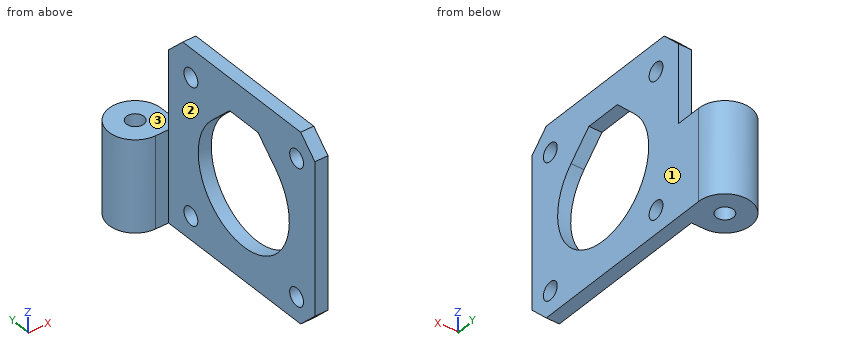
```python
from build123d import *

# Parameters (mm, degrees)
BOX_W        = 2.5
BOX_H        = 36
BOX_DEPTH    = 36
SKETCH_R     = 1.65
PAD_DEPTH    = 17.5
SKETCH001_R  = 1.7
POCKET_DEPTH = 5
CHAMFER_SIZE = 3.5


with BuildPart() as cubo:
    # Box → Box (new body)
    with BuildSketch(Plane.XY):
        with Locations((1.25, 18)):
            Rectangle(BOX_W, BOX_H)
    extrude(amount=BOX_DEPTH)


with BuildPart() as chamfer_body:
    # Sketch → Pad (new body)
    with BuildSketch(Plane.XY):
        with BuildLine():
            Line((0, 0), (2.5, 0))
            Line((2.5, 0), (2.5, 36))
            Line((2.5, 36), (5.000024, 36))
            ThreePointArc((5.000024, 36), (8.535534, 44.535534), (0, 41.000023))
            Line((0, 41.000023), (0, 0))
        make_face()
        with Locations((5, 41)):
            Circle(SKETCH_R, mode=Mode.SUBTRACT)
    extrude(amount=PAD_DEPTH)

    # Fusion: union Cubo
    add(cubo.part)

    # Sketch001 → Pocket (cut)
    with BuildSketch(Plane.YZ.offset(2.5)):
        with Locations((4.5, 30.5)):
            Circle(SKETCH001_R)
        with Locations((30.5, 30.5)):
            Circle(SKETCH001_R)
        with Locations((30.5, 4.5)):
            Circle(SKETCH001_R)
        with Locations((4.5, 4.5)):
            Circle(SKETCH001_R)
        with BuildLine():
            Line((9.580377, 25.419569), (14, 29.839192))
            Line((14, 29.839192), (21, 29.839192))
            Line((21, 29.839192), (25.419623, 25.419569))
            ThreePointArc((9.580377, 25.419569), (17.5, 6.3), (25.419623, 25.419569))
        make_face()
    extrude(amount=-POCKET_DEPTH, mode=Mode.SUBTRACT)

    # Chamfer
    chamfer_edges = [chamfer_body.edges().sort_by_distance(p)[0] for p in [
        (1.25, 36, 36),
        (1.25, 0, 36),
        (1.25, 0, 0),
    ]]
    chamfer(chamfer_edges, length=CHAMFER_SIZE)


with BuildPart() as part_mirroring:
    # Part__Mirroring: instance of Chamfer body
    add(chamfer_body.part.mirror(Plane(origin=(0, 0, 0), x_dir=(0, -1, 0), z_dir=(1, 0, 0))))


solid = part_mirroring.part
```
The listing builds one solid part. Answer for the finished solid, in the listing's coordinates (mm). Face numbers are marked on the shaded views. A direction names the side the tool comes from. Coordinates: 2 decimals unless noted, no trailing zeros. Write each loop counter-clockwise with the first axis right and the second up, starting at its lowest first coordinate (ties: lowest second). Pieces come first, ordered by that corner, then holes. Notation, with made-up numbers: (45, 67.25) -> (99, 67.25) arc R16 ccw to (99, 84.25) -> close; hole circle Ø6 at (87.5, 50.25). An arc over 180 degrees is marked (long way). Write each question's results on one line, items separated by ' | '. Start each with the question number.
1) Straight lines are drawn through the part: probe 1 along Z at (x, y) = (-1.55, 4.5); probe 2 along Z at (x, y) = (-1.95, 17.5); probe 3 along Y at (x, z) = (-1.5, 3.5). For each, find the intervals that lie inside material, in ascending order.
2) A cutting plane is placed at A-A (z = 4.5). Determine the outline of the cut face in (x, y), then the cut area to 3 significant figures.
3) Flat-ended cylindrical pins translate along their axes: pin 1 Ø3 at (x, y) = (-6.5, 40) entering from +Z; pin 2 Ø20 at (y, z) = (17.5, 17.5) entering from +X; pin 3 Ø4.5 at (y, z) = (4.5, 30.5) entering from -X; pin 4 Ø3 at (x, z) = (-0.5, 26) entering from +Y. Find the tip coordinate at first contact, or state that the pin passes through.
4) A cutting plane is placed at C-C (y = 30.5). Determine the outline of the cut face in (x, z), then the cut area to 3 significant figures.
5) A cutting plane is placed at D-D (x = -2). Determine the outline of the cut face in (y, z).
6) A tool of negligible diameter and unlimited length cuts with its end or side. For the marked faces 1, 2 and 3, from which of +Z, -Z, +X, -X, +Y, -Y can it reach the whole face along a straight path? Write none if from no direction.
7) A cutting plane is placed at B-B (z = 14). Determine the outline of the cut face in (x, y).
Values follow:
1) probe 1: 0 to 2.8, 6.2 to 28.8, 32.2 to 36 | probe 2: 0 to 6.3, 29.84 to 36 | probe 3: 0 to 3.13, 5.87 to 29.13, 31.87 to 44.57
2) outline: (-5, 36) -> (-2.5, 36) -> (-2.5, 32.2) -> (0, 32.2) -> (0, 41) arc R5 ccw (long way) to start; (-2.5, 0) -> (0, 0) -> (0, 2.8) -> (-2.5, 2.8) -> close; (-2.5, 6.2) -> (0, 6.2) -> (0, 28.8) -> (-2.5, 28.8) -> close; hole circle Ø3.3 at (-5, 41) | area: 148 mm²
3) pin 1: z = 17.5 | pin 2: through | pin 3: x = -2.5 | pin 4: y = 36
4) outline: (-2.5, 0) -> (0, 0) -> (0, 2.8) -> (-2.5, 2.8) -> close; (-2.5, 6.2) -> (0, 6.2) -> (0, 28.8) -> (-2.5, 28.8) -> close; (-2.5, 32.2) -> (0, 32.2) -> (0, 36) -> (-2.5, 36) -> close | area: 73.0 mm²
5) outline: (0, 3.5) -> (3.5, 0) -> (45, 0) -> (45, 17.5) -> (36, 17.5) -> (36, 32.5) -> (32.5, 36) -> (3.5, 36) -> (0, 32.5) -> close; hole circle Ø3.4 at (4.5, 4.5); hole circle Ø3.4 at (4.5, 30.5); hole (9.58, 25.42) arc R11.2 ccw (long way) to (25.42, 25.42) -> (21, 29.84) -> (14, 29.84) -> close; hole circle Ø3.4 at (30.5, 4.5); hole circle Ø3.4 at (30.5, 30.5)
6) face 1: +Z, -Z, +X, +Y, -Y | face 2: +Z, -Z, -X, -Y | face 3: +Z, +X, -X, +Y
7) outline: (-5, 36) -> (-2.5, 36) -> (-2.5, 28.14) -> (0, 28.14) -> (0, 41) arc R5 ccw (long way) to start; (-2.5, 0) -> (0, 0) -> (0, 6.86) -> (-2.5, 6.86) -> close; hole circle Ø3.3 at (-5, 41)
